Could you check a few things on this model? Use its own coordinates, in mm. Face numbers are marked on the shaded views. A direction names the side the tool comes from. Give positions to 0.01 mm unless a question says otherwise; leave off trailing zeros. Loops run counter-clockwise (first coordinate to the right, second up) from the corner with the lowest first, then second, coordinate; pieces in that order, holes last.
1. Imagine slicing it at D-D (x = -16.5). List the corners of the cut face in (y, z) for me.
2. Imagine slicing it at C-C (z = 72). List the corners of the cut face in (x, y) for me, plus the area to 3 significant figures.
3. Imagine slicing it at B-B (y = -18.75). List the corners of the cut face in (x, z) for me.
4. I need wall thicknesses on line 1 along Z through (x, y) = (1, -15.5); line 2 along Y through (x, z) = (13.5, 45); line 3 along Y through (x, z) = (-5, 11.5). Which ranges of each line are inside material? Lowest first, please.
5. For P1, Ø6, axis at y = -3.5, z = 35, coming from the +X side; P2, Ø5, axis at x = -16.24, y = 9.38, coming from the +Z side; P3, Ø8, axis at x = 9.5, z = 15.5, coming from the -Y side; P4, Ø3, axis at x = 0, y = -18.75, coming from the -Z side, each with a flat end and sliding along its axis, tell me the tip position at first contact or that it passes through.
6. Imagine slicing it at A-A (x = 0). Count the separate pieces of the cut face and the enclosed holes in it, plus the area to 3 significant figures.
7. For the marked faces 1 and 2, which set-ups out of +Z, -Z, +X, -X, +Y, -Y let a thin tool reach every point of the face, with its end or its side?
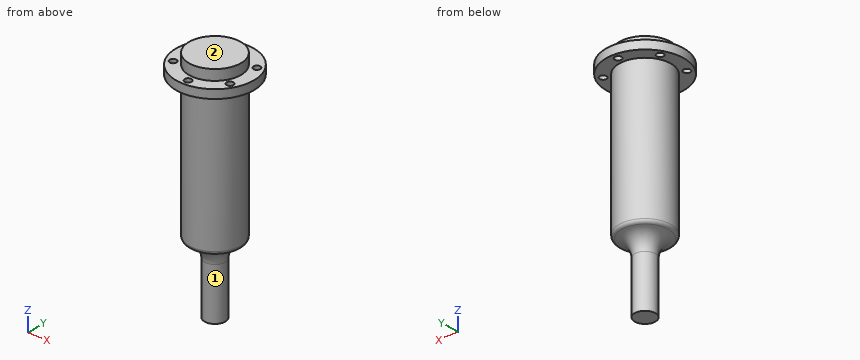
```python
from build123d import *

# Parameters (mm, degrees)
SKETCH1_R             = 15
BOSS_EXTRUDE1_DEPTH   = 77
SKETCH3_R             = 15
SKETCH3_R_2           = 7.5
BOSS_EXTRUDE2_DEPTH   = 17
BOSS_EXTRUDE3_START   = -6
SKETCH4_R             = 22.5
SKETCH4_R_2           = 12.5
SKETCH4_R_3           = 2
BOSS_EXTRUDE3_DEPTH   = 5
SKETCH6_R             = 6
SKETCH6_R_2           = 3
BOSS_EXTRUDE4_DEPTH   = 40
CUT_EXTRUDE2_START    = -72
SKETCH9_R             = 7.5
CUT_EXTRUDE2_DEPTH    = 72
CUT_EXTRUDE3_START    = -5
SKETCH10_R            = 3
CUT_EXTRUDE3_DEPTH    = 5
FILLET1_R             = 10
FILLET2_R             = 2
BOSS_EXTRUDE5_START   = -89
SKETCH12_R            = 7.5
BOSS_EXTRUDE5_DEPTH   = 89
DELETEFACE2_START     = -40
DELETEFACE2_OUTLINE_R = 3
DELETEFACE2_DEPTH     = 45


# Read off the part's stored shape, not the designer's step: DeleteFace2
with BuildPart() as part:
    # Sketch1 → Boss-Extrude1 (new body)
    with BuildSketch(Plane.XY):
        Circle(SKETCH1_R)
    extrude(amount=BOSS_EXTRUDE1_DEPTH)

    # Sketch3 → Boss-Extrude2 (add)
    with BuildSketch(Plane.XY.offset(77)):
        Circle(SKETCH3_R)
        Circle(SKETCH3_R_2, mode=Mode.SUBTRACT)
    extrude(amount=BOSS_EXTRUDE2_DEPTH)

    # Sketch4 → Boss-Extrude3 (add)
    with BuildSketch(Plane.XY.offset(94).offset(BOSS_EXTRUDE3_START)):
        Circle(SKETCH4_R)
        Circle(SKETCH4_R_2, mode=Mode.SUBTRACT)
        with Locations((0, 18.75)):
            Circle(SKETCH4_R_3, mode=Mode.SUBTRACT)
        with Locations((16.237976321, 9.375)):
            Circle(SKETCH4_R_3, mode=Mode.SUBTRACT)
        with Locations((16.237976321, -9.375)):
            Circle(SKETCH4_R_3, mode=Mode.SUBTRACT)
        with Locations((0, -18.75)):
            Circle(SKETCH4_R_3, mode=Mode.SUBTRACT)
        with Locations((-16.237976321, -9.375)):
            Circle(SKETCH4_R_3, mode=Mode.SUBTRACT)
        with Locations((-16.237976321, 9.375)):
            Circle(SKETCH4_R_3, mode=Mode.SUBTRACT)
    extrude(amount=-BOSS_EXTRUDE3_DEPTH)

    # Sketch6 → Boss-Extrude4 (add)
    with BuildSketch(Plane(origin=(0, 0, 0), x_dir=(-1, 0, 0), z_dir=(0, 0, -1))):
        with Locations(Location((0, 0, 0), (0, 0, 180))):
            Circle(SKETCH6_R)
        Circle(SKETCH6_R_2, mode=Mode.SUBTRACT)
    extrude(amount=BOSS_EXTRUDE4_DEPTH)

    # Sketch9 → Cut-Extrude2 (cut)
    with BuildSketch(Plane.XY.offset(77).offset(CUT_EXTRUDE2_START)):
        Circle(SKETCH9_R)
    extrude(amount=CUT_EXTRUDE2_DEPTH, mode=Mode.SUBTRACT)

    # Sketch10 → Cut-Extrude3 (cut)
    with BuildSketch(Plane(origin=(0, 0, 0), x_dir=(-1, 0, 0), z_dir=(0, 0, -1)).offset(CUT_EXTRUDE3_START)):
        with Locations(Location((0, 0, 0), (0, 0, 180))):
            Circle(SKETCH10_R)
    extrude(amount=CUT_EXTRUDE3_DEPTH, mode=Mode.SUBTRACT)

    # Fillet1
    # the kernel refuses this fillet: 10 mm, written as the material it adds along each edge
    with BuildSketch(Plane(origin=(0, 0, 0), x_dir=(1, 0, 0), z_dir=(0, 1, 0))) as fillet1_piece_1:
        with BuildLine():
            CenterArc((16, 9.949874371), FILLET1_R, 180, 84.260829523)
            Line((6, 9.949874371), (5.8, 9.949874371))
            Line((5.8, 9.949874371), (5.8, 0))
            Line((5.8, 0), (6, -0.2))
            ThreePointArc((6, -0.2), (10.5, -0.2), (14.98, -0.198997487))
            Line((14.98, -0.198997487), (15, 0))
        make_face()
    revolve(axis=Axis((0, 0, 0), (0, 0, -1)))

    # Fillet2
    fillet2_edges = [part.edges().sort_by_distance(p)[0] for p in [
        (-15, 0, 0),
    ]]
    fillet(fillet2_edges, radius=FILLET2_R)

    # Sketch12 → Boss-Extrude5 (add)
    with BuildSketch(Plane.XY.offset(94).offset(BOSS_EXTRUDE5_START)):
        Circle(SKETCH12_R)
    extrude(amount=BOSS_EXTRUDE5_DEPTH)

    # DeleteFace2 outline → DeleteFace2 (add)
    with BuildSketch(Plane.XY.offset(DELETEFACE2_START)):
        Circle(DELETEFACE2_OUTLINE_R)
    extrude(amount=DELETEFACE2_DEPTH)


solid = part.part
```
Derived:
1. outline: (-15.3, 83) - (-11.36, 83) - (-11.36, 88) - (-15.3, 88) - close; (-7.39, 83) - (7.39, 83) - (7.39, 88) - (-7.39, 88) - close; (11.36, 83) - (15.3, 83) - (15.3, 88) - (11.36, 88) - close
2. outline: circle Ø30 at (0, 0)
2. area: 707 mm2
3. outline: (-12.44, 83) - (-2, 83) - (-2, 88) - (-12.44, 88) - close; (2, 83) - (12.44, 83) - (12.44, 88) - (2, 88) - close
4. line 1: z = 83 to 88
4. line 2: y = -6.54 to 6.54
4. line 3: y = -14.14 to 14.14
5. P1: stops at x = 14.99
5. P2: stops at z = 88
5. P3: stops at y = -13.96
5. P4: passes through
6. separate pieces: 3
6. enclosed holes: 0
6. area: 3,380 mm2
7. face 1: -Z
7. face 2: +Z, +X, -X, +Y, -Y
